The listing builds one solid part. Answer for the finished solid, in the listing's coordinates (mm). Face numbers are marked on the shaded views. A direction names the side the tool comes from. Give positions to 0.01 mm unless a question says otherwise; leave off trailing zeros. Order: outer loops, then holes, each group sorted by start corner. A loop starts at its lowest first (then second) coordinate and runs counter-clockwise, first axis right, second up. Notation, with made-up numbers: (-5.75, -10) - (46.25, -10) arc R23 ccw to (46.25, 10) - close; hole circle Ø2 at (31.5, 49.25). An arc over 180 degrees is marked (long way). Answer in a Markdown table with one row per item.
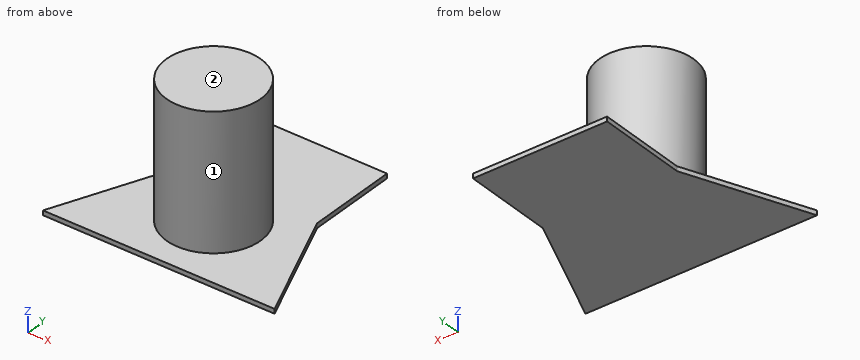
from build123d import *

# Parameters (mm, degrees)
EXTRUDE_1_DEPTH = 2
SKETCH_3_R      = 20.333518405
EXTRUDE_2_DEPTH = 60


with BuildPart() as part:
    # 草图1 → 凸台-拉伸1 (new body)
    with BuildSketch(Plane.XY):
        Polygon((-50, 0), (-28.960949348, 50.922075999), (-28.960949348, 90), (28.960949348, 90), (28.960949348, 50.922075999), (50, 0), align=None)
    extrude(amount=EXTRUDE_1_DEPTH)

    # 草图3 → 凸台-拉伸2 (add)
    with BuildSketch(Plane(origin=(0, 0, 0), x_dir=(-1, 0, 0), z_dir=(0, 0, -1))):
        with Locations((0, 30.596151571)):
            Circle(SKETCH_3_R)
    extrude(amount=-EXTRUDE_2_DEPTH)


solid = part.part
Item 1: Each of these flat-tipped pins is pushed along its axis until it touches: P1, Ø1, axis at y = 19.5, z = 52.5, coming from the +X side; P2, Ø6, axis at y = 46, z = 40, coming from the -X side; P3, Ø1, axis at x = -12.5, z = 21.5, coming from the +Y side; P4, Ø4, axis at x = -23.5, z = 41.5, coming from the +Y side. Where does it stop, or does it pass through?
Answer block:
| item | result |
|---|---|
| P1 | x = 17.35 |
| P2 | x = -16.11 |
| P3 | y = 47.01 |
| P4 | through |
Item 2: Find section C-C on z = 4. Write down the section's boundary in (x, y).
Answer block:
| item | result |
|---|---|
| outline | circle Ø40.67 at (0, 30.6) |
Item 3: Find section B-B on y = 40. Write down the section's boundary in (x, z), then the cut area to 3 significant figures.
Answer block:
| item | result |
|---|---|
| outline | (-33.47, 0) - (33.47, 0) - (33.47, 2) - (18.03, 2) - (18.03, 60) - (-18.03, 60) - (-18.03, 2) - (-33.47, 2) - close |
| area | 2,230 mm² |
Item 4: Find section A-A on x = 0. Write down the section's boundary in (y, z), then the cut area to 3 significant figures.
Answer block:
| item | result |
|---|---|
| outline | (0, 0) - (90, 0) - (90, 2) - (50.93, 2) - (50.93, 60) - (10.26, 60) - (10.26, 2) - (0, 2) - close |
| area | 2,540 mm² |
Item 5: Which of the six approach directions +Z, -Z, +X, -X, +Y, -Y give full straight-line access (tool end or side, diameter ignored) to the marked faces 1 and 2?
Answer block:
| item | result |
|---|---|
| face 1 | +Z |
| face 2 | +Z, +X, -X, +Y, -Y |
Item 6: Find section D-D on y = 83. Write down the section's boundary in (x, z).
Answer block:
| item | result |
|---|---|
| outline | (-28.96, 0) - (28.96, 0) - (28.96, 2) - (-28.96, 2) - close |
Item 7: Consider line 1 (Z direction, x = -20.5, y = 38); line 2 (X direction, y = 49, z = 50.5); line 3 (Y direction, x = -7, z = 36). Determine where each line is inside the solid, lowest interval first.
Answer block:
| item | result |
|---|---|
| line 1 | 0 to 2 |
| line 2 | -8.65 to 8.65 |
| line 3 | 11.51 to 49.69 |
